Could you check a few things on this drawing? It's one solid part, dimensions in mm from its lowest x, y, z. A direction names the side the tool comes from. Give positions to 0.01 mm unless a question says otherwise; leave off trailing zeros. Loops run counter-clockwise (first coordinate to the right, second up) from the corner with the lowest first, then second, coordinate; pieces in that order, holes last. Notation, with made-up numbers: (50.5, -29) - (98.5, -29) arc R23 cw to (98.5, -3) - close; hole circle Ø5 at (-24, 38). An arc over 180 degrees is marked (long way). Return JSON: item names as keys, results as strings. Group by question number.
(1) On a 3-axis mill with a long thin cutter (end or side, diameter ignored), from which of +Z, -Z, +X, -X, +Y, -Y can I reach the whole of each face in a straight line? I mean the marked faces 4 and 5. Say none if no direction works.
(2) If we section it at C-C (z = 3.45): Please give me the cut outline in (x, y).
(3) If we section it at D-D (x = 4.75): Please give me the cut outline in (y, z).
(4) If we mould it in two halves opening along X, with no side actions, what happens to the marked faces 1, 2 and 3? For each: released by +X, released by -X, zero draft, split by the parting line, or undercut.
(5) For P1, Ø1, axis at x = 2, z = 4, coming from the -Y side, with a flat end and sliding along its axis, tell me the tip position at first contact or that it passes through.
(6) If we section it at A-A (y = 1.5): Please give me the cut outline in (x, z).
(7) I need wall thicknesses on probe 1 along Z at (x, y) = (2.75, 1.7); probe 2 along X at (y, z) = (1.1, 3.85); probe 3 along X at (y, z) = (0.7, 3.3). Which ranges of each line are inside material? Lowest first, please. Write a range as [from, to].
(8) If we section it at B-B (x = 1.65): Please give me the cut outline in (y, z), then the cut area to 3 significant figures.
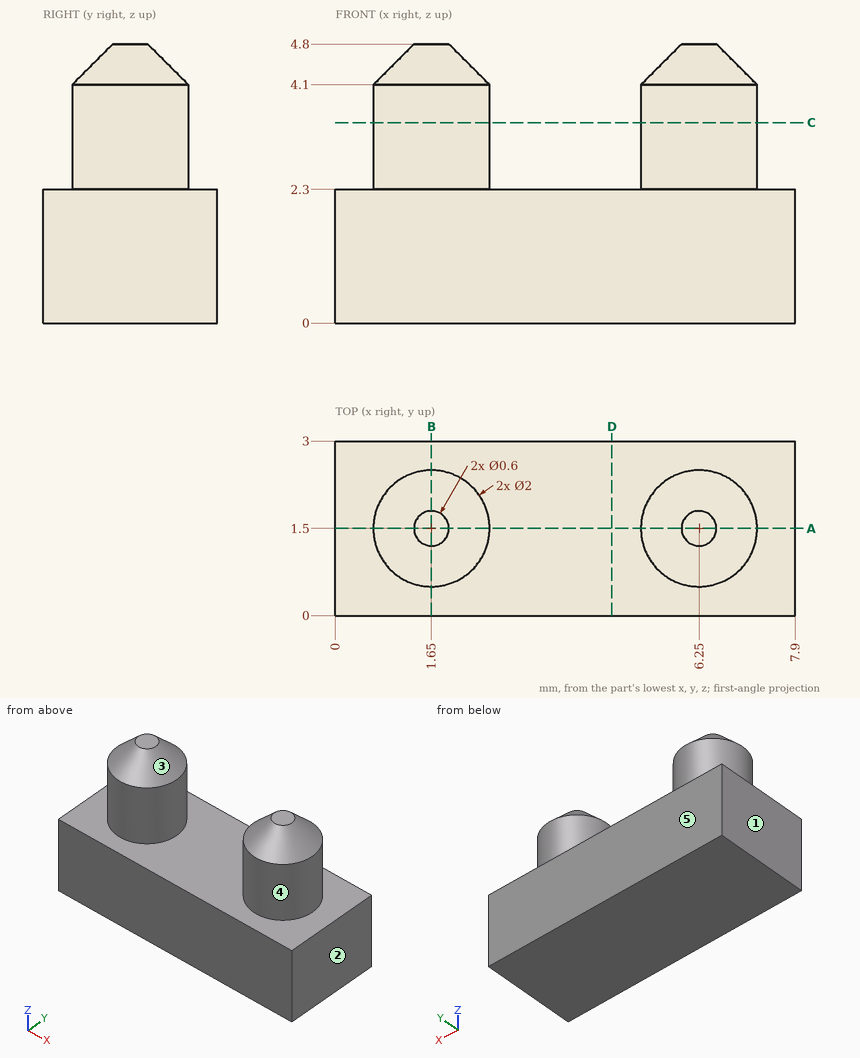
Values:
{
 "1": {"face 4": "+Z", "face 5": "+Z, -Z, +X, -X, +Y"},
 "2": {"outline": "circle Ø2 at (1.65, 1.5); circle Ø2 at (6.25, 1.5)"},
 "3": {"outline": "(0, 0) - (3, 0) - (3, 2.3) - (0, 2.3) - close"},
 "4": {"face 1": "released by -X", "face 2": "released by +X", "face 3": "undercut"},
 "5": {"P1": "y = 0.5"},
 "6": {"outline": "(0, 0) - (7.9, 0) - (7.9, 2.3) - (7.25, 2.3) - (7.25, 4.1) - (6.55, 4.8) - (5.95, 4.8) - (5.25, 4.1) - (5.25, 2.3) - (2.65, 2.3) - (2.65, 4.1) - (1.95, 4.8) - (1.35, 4.8) - (0.65, 4.1) - (0.65, 2.3) - (0, 2.3) - close"},
 "7": {"probe 1": "[0, 2.3]", "probe 2": "[0.73, 2.57], [5.33, 7.17]", "probe 3": "[1.05, 2.25], [5.65, 6.85]"},
 "8": {"outline": "(0, 0) - (3, 0) - (3, 2.3) - (2.5, 2.3) - (2.5, 4.1) - (1.8, 4.8) - (1.2, 4.8) - (0.5, 4.1) - (0.5, 2.3) - (0, 2.3) - close", "area": "11.4 mm2"}
}
